```python
from build123d import *

# Parameters (mm, degrees)
F0_R     = 50.8204008134
F1_DEPTH = 12.7
F1_TAPER = 3
F3_DEPTH = 25
F4_R     = 5


with BuildPart() as f1:
    # F0 (on Top) → F1 (new body)
    with BuildSketch(Plane.XY):
        Circle(F0_R)
    extrude(amount=F1_DEPTH, taper=F1_TAPER)

    # F2 (on face) → F3 (join)
    with BuildSketch(Plane.XY.offset(12.7)):
        with BuildLine():
            ThreePointArc((-10.3685208828, -35.279545933), (-11.5330508003, -31.1117961239), (-14.6893061002, -28.1513365513))
            ThreePointArc((-14.6893061002, -28.1513365513), (-25.2845296612, -39.4472957421), (-10.3685208828, -35.279545933))
        make_face()
        with BuildLine():
            ThreePointArc((46.1865502421, 0), (37.1504314244, 9.0361188178), (28.1143126066, 0))
            ThreePointArc((28.1143126066, 0), (37.1504314244, -9.0361188178), (46.1865502421, 0))
        make_face()
        with BuildLine():
            ThreePointArc((-22.1275595237, 27.55375579), (-33.8414364746, 29.8480310368), (-23.8585792296, 23.3042421225))
            ThreePointArc((-23.8585792296, 23.3042421225), (-22.5769153544, 25.2594805432), (-22.1275595237, 27.55375579))
        make_face()
    extrude(amount=-F3_DEPTH)

    # F4
    f4_edges = [f1.edges().sort_by_distance(p)[0] for p in [
        (-50.154822, 0, 12.7),
    ]]
    fillet(f4_edges, radius=F4_R)


solid = f1.part
```
Work out the finished part from the listing and answer in its coordinate system (mm). A direction names the side the tool comes from. Round coordinates to 2 decimals unless told otherwise and drop trailing zeros. Loops run counter-clockwise (first coordinate to the right, second up) from the corner with the lowest first, then second, coordinate; pieces in that order, holes last. Notation, with made-up numbers: (-10.75, -11) -> (21.25, -11) arc R20 ccw to (21.25, -1) -> close; hole circle Ø7 at (8.5, 39.25). An arc over 180 degrees is marked (long way). Write each question's results on one line, items separated by ' | '. Start each with the question number.
1. Section B-B (z = 6.5) is taken. Determine the outline of the cut face in (x, y), plus the area to 3 significant figures.
2. Given pin 1 Ø10 at (x, y) = (40.5, 12.5) entering from -Z; pin 2 Ø6 at (x, z) = (-12, -1) entering from +Y; pin 3 Ø2 at (y, z) = (26, 8.5) entering from -X; pin 4 Ø12 at (x, z) = (-21, 9.5) entering from -Y, each flat-ended and moving along its own axis, determine where each tip first touches the part or whether it passes through.
3. Find the intervals of material crossed by probe 1 along Z at (x, y) = (-23, -25); probe 2 along Y at (x, z) = (-24.5, -9.75); probe 3 along Y at (x, z) = (10, 3), in increasing order. Write a range as from..to.
4. A tool of negligible diameter and unlimited length cuts with its end or side. For faces 1 (the face through (-1, 1, 12.7)), 2 (the face through (-1, 1, 0)), from which of +Z, -Z, +X, -X, +Y, -Y can it reach the whole face along a straight path? Write none if from no direction.
5. Section A-A (x = 0) is taken. Determine the outline of the cut face in (y, z).
Evaluation:
1) outline: circle Ø100.96 at (0, 0) | area: 8,010 mm2
2) pin 1: stops at z = -12.3 | pin 2: stops at y = 49.99 | pin 3: stops at x = -43.72 | pin 4: stops at y = -48.06
3) probe 1: z = 0..12.7 | probe 2: y = -40.53..-30.03, 22.73..32.37 | probe 3: y = -49.67..49.67
4) face 1: +Z, +X, -X, +Y, -Y | face 2: -Z
5) outline: (-50.82, 0) -> (50.82, 0) -> (50.4, 7.96) arc R5 ccw to (45.41, 12.7) -> (-45.41, 12.7) arc R5 ccw to (-50.4, 7.96) -> close
